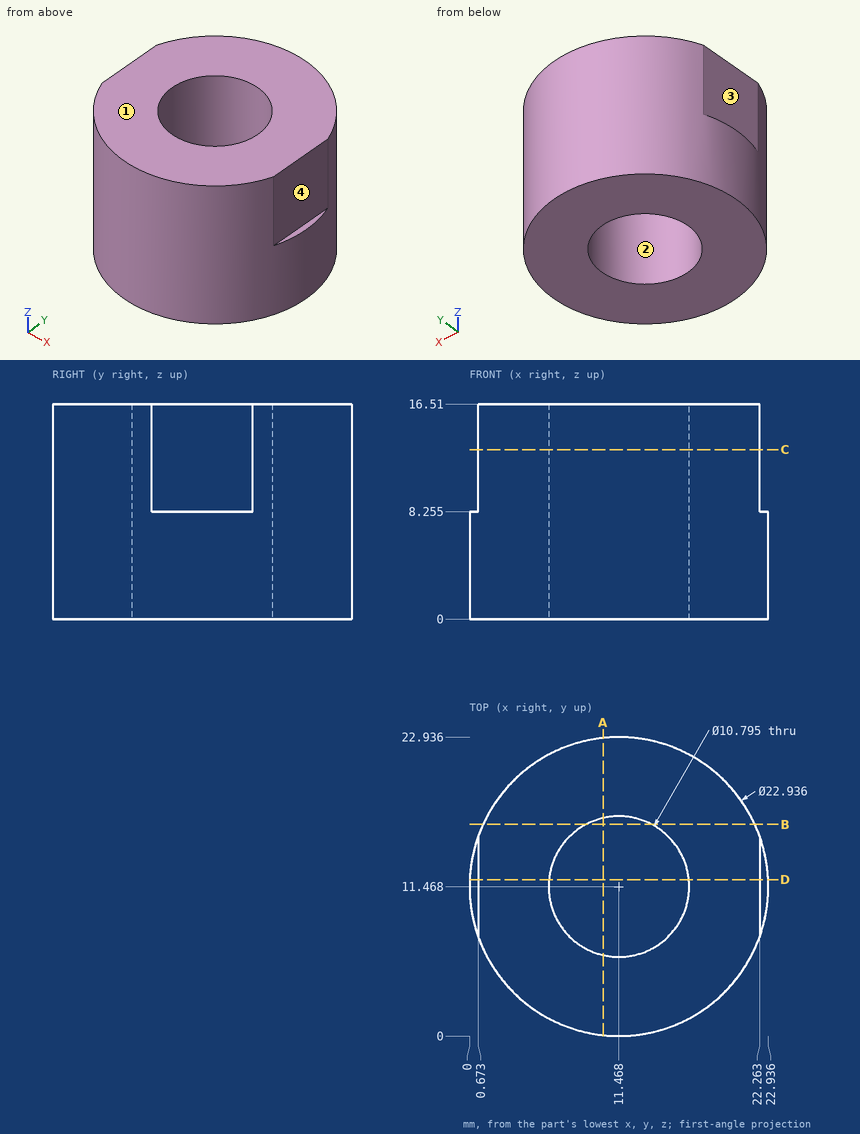
Check sheet for the drawn part. Datum: minimum x, y, z corner. Units: mm. Round coordinates to 2 decimals unless told otherwise and drop trailing zeros. Loops run counter-clockwise (first coordinate to the right, second up) from the corner with the lowest first, then second, coordinate; pieces in that order, holes last. Notation, with made-up numbers: (-26, -12) - (1, -12) arc R25 cw to (1, 4) - close; hole circle Ø8 at (36.5, -18.75). An arc over 180 degrees is marked (long way). Answer as a JSON object with one key per item and string values. Group by question number.
Q1. Gauge pin test, flat ends, axial feed: P1, Ø2, axis at x = 16.5, z = 11, coming from the -Y side; P2, Ø10, axis at x = 19.5, y = 7, coming from the -Z side; P3, Ø1, axis at x = 9, z = 10, coming from the -Y side; P4, Ø1, axis at x = 5, z = 6.5, coming from the -Y side (1 decimal). Record the tip position at first contact, or that the pin passes through.
Q2. Scan lines: line 1 along Y through (x, z) = (11.25, 9) (1 decimal); line 2 along X through (y, z) = (11.5, 15.25); line 3 along Y through (x, z) = (9.25, 5.5). Record each from-to range of solid material in increasing order. Write a range as [from, to].
Q3. Sectioned sample at D-D, the plane y = 12. Enter the section's corners in (x, z) (1 decimal).
Q4. Sectioned sample at B-B, the plane y = 16.25. Enter the section's corners in (x, z) (1 decimal).
Q5. Sectioned sample at A-A, the plane x = 10.25. Enter the section's corners in (y, z) (1 decimal).
Q6. Mould release check, pull along X, two halves, no side actions. Record for the marked faces 1, 2, 3 and 4: released by +X, released by -X, zero draft, split by the parting line, or undercut.
Q7. Sectioned sample at C-C, the plane z = 13. Enter the section's corners in (x, y) (1 decimal), plus the area to 3 significant figures.
Solution:
{
 "1": {"P1": "stops at y = 0.73", "P2": "stops at z = 0", "P3": "stops at y = 0.17", "P4": "stops at y = 1.7"},
 "2": {"line 1": "y = [0, 6.1], [16.9, 22.9]", "line 2": "x = [0.67, 6.07], [16.87, 22.26]", "line 3": "y = [0.22, 6.55], [16.39, 22.72]"},
 "3": {"outline": "(0, 0) - (6.1, 0) - (6.1, 16.5) - (0.7, 16.5) - (0.7, 8.3) - (0, 8.3) - close; (16.8, 0) - (22.9, 0) - (22.9, 8.3) - (22.3, 8.3) - (22.3, 16.5) - (16.8, 16.5) - close"},
 "4": {"outline": "(1, 0) - (9, 0) - (9, 16.5) - (1, 16.5) - close; (14, 0) - (21.9, 0) - (21.9, 16.5) - (14, 16.5) - close"},
 "5": {"outline": "(0.1, 0) - (6.2, 0) - (6.2, 16.5) - (0.1, 16.5) - close; (16.7, 0) - (22.9, 0) - (22.9, 16.5) - (16.7, 16.5) - close"},
 "6": {"face 1": "zero draft", "face 2": "undercut", "face 3": "released by -X", "face 4": "released by +X"},
 "7": {"outline": "(0.7, 7.6) arc R11.5 ccw to (22.3, 7.6) - (22.3, 15.3) arc R11.5 ccw to (0.7, 15.3) - close; hole circle Ø10.8 at (11.5, 11.5)", "area": "315 mm²"}
}
